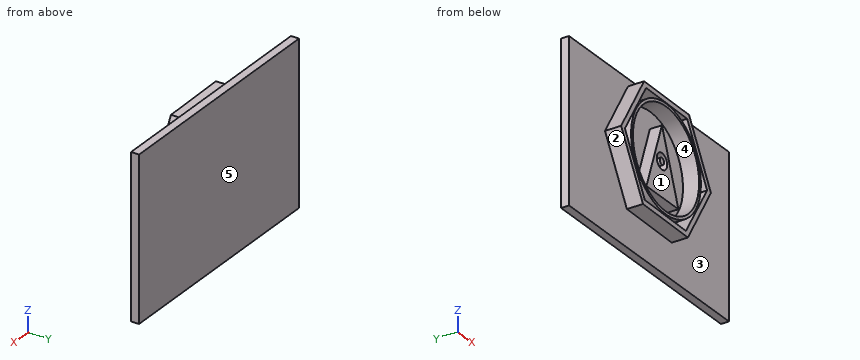
```python
from build123d import *

# Parameters (mm, degrees)
F0_W     = 150
F0_H     = 100
F1_DEPTH = 5
F2_R     = 4.890759
F2_R_2   = 2.063012
F3_DEPTH = 7.5
F5_DEPTH = 10
F6_R     = 32.750656
F6_R_2   = 31.034289
F7_DEPTH = 10


with BuildPart() as f1:
    # F0 (on Front) → F1 (new body)
    with BuildSketch(Plane.XZ):
        with Locations((-0.814352, 12.874251)):
            Rectangle(F0_W, F0_H)
    extrude(amount=F1_DEPTH)

    # F2 (on face) → F3 (join)
    with BuildSketch(Plane.XZ.offset(5)):
        Polygon((0, 42.534135), (-14.594158, 0), (15.405842, 0), align=None)
        with Locations((0, 21.267068)):
            Circle(F2_R, mode=Mode.SUBTRACT)
        with Locations((0, 21.267068)):
            Circle(F2_R_2)
    extrude(amount=F3_DEPTH)

    # F4 (on face) → F5 (join)
    with BuildSketch(Plane.XZ.offset(5)):
        Polygon((-20.528079, 58.401592), (-42.103289, 22.241354), (-21.57521, -14.523444), (20.528079, -15.128005), (42.103289, 21.032233), (21.57521, 57.797031), align=None)
        Polygon((-19.871907, -11.400712), (-38.547273, 22.327617), (-18.675366, 55.365123), (19.871907, 54.674299), (38.547273, 20.94597), (18.675366, -12.091536), align=None, mode=Mode.SUBTRACT)
    extrude(amount=F5_DEPTH)

    # F6 (on face) → F7 (join)
    with BuildSketch(Plane.XZ.offset(5)):
        with Locations((0, 21.882644)):
            Circle(F6_R)
        with Locations((0, 21.882644)):
            Circle(F6_R_2, mode=Mode.SUBTRACT)
    extrude(amount=F7_DEPTH)


solid = f1.part
```
The model under review builds one solid part; all positions refer to its coordinate system, in mm. Face numbers are marked on the shaded views. A direction names the side the tool comes from. Round coordinates to 2 decimals unless told otherwise and drop trailing zeros. Loops run counter-clockwise (first coordinate to the right, second up) from the corner with the lowest first, then second, coordinate; pieces in that order, holes last. Notation, with made-up numbers: M 30,43.25 L 35,43.25 A12 ccw 35,61.25 Z; hole C 12.5,25.5 d1. An arc over 180 degrees is marked long. Answer as a JSON object with one key per item and string values.
(1) Take a section at C-C on z = -28. Give the boundary of the cut face in (x, y).
Resolved:
{"outline": "M -75.81,-5 L 74.19,-5 L 74.19,0 L -75.81,0 Z"}
(2) Draft analysis for pull direction X (two halves, no side actions). For the marked faces 1, 2 and 3, state which applies: released by +X, released by -X, zero draft, split by the parting line, or undercut.
Resolved:
{"face 1": "undercut", "face 2": "released by -X", "face 3": "zero draft"}
(3) Tool access review of the marked faces 4 and 5: name each direction out of +Z, -Z, +X, -X, +Y, -Y from which nothing blocks a thin tool from reaching the whole face with its end or side.
Resolved:
{"face 4": "-Y", "face 5": "+Z, -Z, +X, -X, +Y"}
(4) Take a section at A-A on z = 29. Give the boundary of the cut face in (x, y).
Resolved:
{"outline": "M -75.81,-5 L -38.07,-5 L -38.07,-15 L -34.53,-15 L -34.53,-5 L -31.97,-5 L -31.97,-15 L -30.21,-15 L -30.21,-5 L -4.64,-5 L -4.64,-12.5 L 4.9,-12.5 L 4.9,-5 L 30.21,-5 L 30.21,-15 L 31.97,-15 L 31.97,-5 L 34.09,-5 L 34.09,-15 L 37.65,-15 L 37.65,-5 L 74.19,-5 L 74.19,0 L -75.81,0 Z"}
(5) Clearance check with flat-ended pins moving along their axes: P1, Ø24, axis at x = -3, z = 15.5, coming from the -Y side; P2, Ø4, axis at y = -10.5, z = 22, coming from the +X side; P3, Ø6, axis at x = 8, y = -9.5, coming from the -Z side. State where each tip first meets the part, or that it passes through.
Resolved:
{"P1": "y = -12.5", "P2": "x = 42.1", "P3": "z = -14.99"}
(6) Take a section at B-B on x = 51. Give the boundary of the cut face in (y, z), and give its area (3 significant figures).
Resolved:
{"outline": "M -5,-37.13 L 0,-37.13 L 0,62.87 L -5,62.87 Z", "area": "500 mm²"}
(7) To check wall thickness, follow line 1 along X through (y, z) = (-5.25, 14.5); line 2 along X through (y, z) = (-6, 6); line 3 along Z through (x, y) = (26.5, -8.75). State the ranges of each line that lie inside material, in increasing order.
Resolved:
{"line 1": "-37.78 to -34.21, -31.91 to -30.14, -9.62 to 10.15, 30.14 to 31.91, 34.67 to 38.21", "line 2": "-33.03 to -29.51, -28.64 to -26.66, -12.54 to 13.23, 26.66 to 28.64, 29.56 to 33.13", "line 3": "-5.12 to 0.92, 2.64 to 5.73, 38.03 to 41.13, 42.7 to 48.98"}
